Part model, mm, in its own coordinate system. A direction names the side the tool comes from. Give positions to 0.01 mm unless a question says otherwise; leave off trailing zeros. Order: outer loops, then holes, each group sorted by start corner. A loop starts at its lowest first (then second) coordinate and runs counter-clockwise, first axis right, second up. Notation, with made-up numbers: (-28.75, 25.25) -> (-17.75, 25.25) arc R17 cw to (-17.75, 38.25) -> close; hole circle Ø3 at (-17, 87). An arc over 180 degrees is marked (long way). Write item = value, one per line. Start each with the question number.
Item 1: Tool access for faces 1 (the face through (14.234, 5, -19)), 2 (the face through (3.234, 5, -18)), 3 (the face through (8.4, 10, -18.8)): list every direction of +Z, -Z, +X, -X, +Y, -Y with a clear straight run to the whole face (end or side of a thin tool).
Item 2: Pull direction Z, two halves, no side cores. Call faces 4 (the face through (-9, 5, 46.719)), 5 (the face through (-31.616, 5, -18)), 6 (the face through (27.234, 5, 75)): +Z half, -Z half, draft (parallel to the pull), parting line (faces both ways), or undercut.
Item 3: Band-saw the part on D-D on z = -92.5. Write the cut outline in (x, y).
Item 4: Flat gauge pins, fed straight in: P1, Ø2, axis at x = -2, y = 4.5, coming from the -Z side; P2, Ø3, axis at x = 25, y = 7.5, coming from the +Z side; P3, Ø5, axis at y = 3.5, z = -112, coming from the -X side; P4, Ø2, axis at x = -38.72, z = 42.03, coming from the +Y side. Where does each tip first touch, or does it go through?
Item 5: Band-saw the part on A-A on x = -17.5. Write the cut outline in (y, z).
Item 6: Band-saw the part on B-B on z = -62. Write the cut outline in (x, y), plus the area to 3 significant figures.
Item 7: Band-saw the part on C-C on y = 3.5. Write the cut outline in (x, z).
Item 8: Drill centre lines: line 1 along X through (y, z) = (8.75, -61.5); line 2 along Z through (x, y) = (20, 2.25); line 3 along Z through (x, y) = (22.5, 6.75). Where is each one in solid material? Low to high.
```python
from build123d import *

# Parameters (mm, degrees)
SKETCH1_R           = 1.7
SKETCH1_W           = 30
SKETCH1_H           = 100
BOSS_EXTRUDE1_DEPTH = 10


with BuildPart() as part:
    # Sketch1 → Boss-Extrude1 (new body)
    with BuildSketch(Plane(origin=(0, 0, 0), x_dir=(1, 0, 0), z_dir=(0, 1, 0))):
        Polygon((32.234241277, 138.28125), (32.234241277, 68.28125), (14.234241277, 68.28125), (14.234241277, -31.71875), (32.234241277, -31.71875), (32.234241277, -101.71875), (27.234241277, -101.71875), (27.234241277, -46.71875), (-30.265758723, -46.71875), (-44.162144835, -46.71875), (-44.162144835, 83.28125), (-30.265758723, 83.28125), (27.234241277, 83.28125), (27.234241277, 138.28125), align=None)
        with Locations((22.234241277, 74.963265867)):
            Circle(SKETCH1_R, mode=Mode.SUBTRACT)
        with Locations((22.234241277, -38.400765867)):
            Circle(SKETCH1_R, mode=Mode.SUBTRACT)
        with Locations((-38.719051078, -42.025453022)):
            Circle(SKETCH1_R, mode=Mode.SUBTRACT)
        with Locations((-38.719051078, 78.587953022)):
            Circle(SKETCH1_R, mode=Mode.SUBTRACT)
        with Locations((-11.765758723, 18.28125)):
            Rectangle(SKETCH1_W, SKETCH1_H, mode=Mode.SUBTRACT)
        with BuildLine():
            Line((-31.615758723, 18.28125), (-31.615758723, 68.28125))
            ThreePointArc((-31.615758723, 68.28125), (-30.265758723, 69.63125), (-28.915758723, 68.28125))
            Line((-28.915758723, 68.28125), (-28.915758723, 18.28125))
            Line((-28.915758723, 18.28125), (-28.915758723, -31.71875))
            ThreePointArc((-28.915758723, -31.71875), (-30.265758723, -33.06875), (-31.615758723, -31.71875))
            Line((-31.615758723, -31.71875), (-31.615758723, 18.28125))
        make_face(mode=Mode.SUBTRACT)
        with BuildLine():
            Line((5.384241277, 18.28125), (5.384241277, 68.28125))
            ThreePointArc((5.384241277, 68.28125), (6.734241277, 69.63125), (8.084241277, 68.28125))
            Line((8.084241277, 68.28125), (8.084241277, 18.28125))
            Line((8.084241277, 18.28125), (8.084241277, -31.71875))
            ThreePointArc((8.084241277, -31.71875), (6.734241277, -33.06875), (5.384241277, -31.71875))
            Line((5.384241277, -31.71875), (5.384241277, 18.28125))
        make_face(mode=Mode.SUBTRACT)
    extrude(amount=BOSS_EXTRUDE1_DEPTH)


solid = part.part
```
Values found:
q1.face_1 = +X, +Y, -Y
q1.face_2 = +Y, -Y
q1.face_3 = +Z, -Z, +X, -X, +Y
q2.face_4 = +Z half
q2.face_5 = undercut
q2.face_6 = draft
q3.outline = (27.23, 0) -> (32.23, 0) -> (32.23, 10) -> (27.23, 10) -> close
q4.P1 = -83.28
q4.P2 = 46.72
q4.P3 = 27.23
q4.P4 = through
q5.outline = (0, -83.28) -> (10, -83.28) -> (10, -68.28) -> (0, -68.28) -> close; (0, 31.72) -> (10, 31.72) -> (10, 46.72) -> (0, 46.72) -> close
q6.outline = (-44.16, 0) -> (-31.62, 0) -> (-31.62, 10) -> (-44.16, 10) -> close; (-28.92, 0) -> (-26.77, 0) -> (-26.77, 10) -> (-28.92, 10) -> close; (3.23, 0) -> (5.38, 0) -> (5.38, 10) -> (3.23, 10) -> close; (8.08, 0) -> (14.23, 0) -> (14.23, 10) -> (8.08, 10) -> close
q6.area = 230 mm^2
q7.outline = (-44.16, -83.28) -> (27.23, -83.28) -> (27.23, -138.28) -> (32.23, -138.28) -> (32.23, -68.28) -> (14.23, -68.28) -> (14.23, 31.72) -> (32.23, 31.72) -> (32.23, 101.72) -> (27.23, 101.72) -> (27.23, 46.72) -> (-44.16, 46.72) -> close; hole circle Ø3.4 at (-38.72, -78.59); hole circle Ø3.4 at (-38.72, 42.03); hole (-31.62, -68.28) arc R1.35 ccw to (-28.92, -68.28) -> (-28.92, 31.72) arc R1.35 ccw to (-31.62, 31.72) -> close; hole (-26.77, -68.28) -> (3.23, -68.28) -> (3.23, 31.72) -> (-26.77, 31.72) -> close; hole (5.38, -68.28) arc R1.35 ccw to (8.08, -68.28) -> (8.08, 31.72) arc R1.35 ccw to (5.38, 31.72) -> close; hole circle Ø3.4 at (22.23, -74.96); hole circle Ø3.4 at (22.23, 38.4)
q8.line_1 = -44.16 to -31.62, -28.92 to -26.77, 3.23 to 5.38, 8.08 to 14.23
q8.line_2 = -83.28 to -68.28, 31.72 to 46.72
q8.line_3 = -83.28 to -76.64, -73.28 to -68.28, 31.72 to 36.72, 40.08 to 46.72
